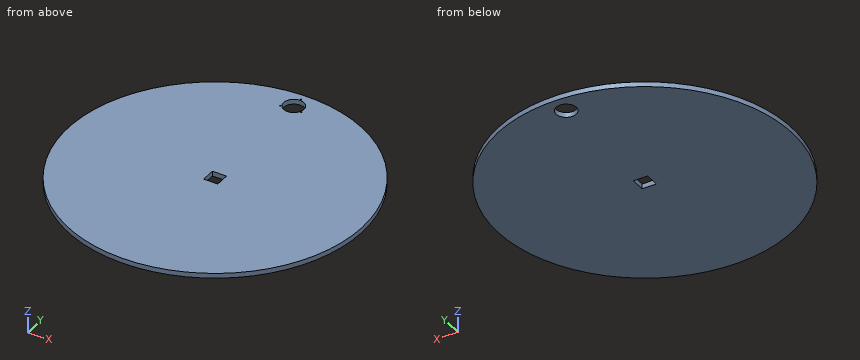
```python
from build123d import *

# Parameters (mm, degrees)
F0_R     = 600
F0_W     = 58.1
F0_H     = 58.1
F1_DEPTH = 20
F3_R     = 41.5
F4_DEPTH = 20.001
F5_D     = 5.1054
F5_DEPTH = 15.81
F5_TIP   = 1.5338169022


with BuildPart() as f1:
    # F0 (on Top) → F1 (new body)
    with BuildSketch(Plane.XY):
        Circle(F0_R)
        Rectangle(F0_W, F0_H, mode=Mode.SUBTRACT)
    extrude(amount=F1_DEPTH)

    # F3 (on offset) → F4 (cut, through all)
    with BuildSketch(Plane.XY.offset(20)):
        with Locations((0.1939173973, 525.9999642548)):
            Circle(F3_R)
    extrude(amount=-F4_DEPTH, mode=Mode.SUBTRACT)

    # F5
    with Locations(Plane.XY.offset(20)):
        with Locations((-40.7258506305, 502.1913310914), (43.0168926358, 505.8476182242), (0.1938496983, 573.0663310914)):
            Hole(F5_D / 2, depth=F5_DEPTH)
            with Locations((0, 0, -(F5_DEPTH + F5_TIP / 2))):  # 118° drill point
                Cone(0, F5_D / 2, F5_TIP, mode=Mode.SUBTRACT)


solid = f1.part
```
Could you check a few things on this model? Use its own coordinates, in mm. Coordinates: 2 decimals unless noted, no trailing zeros. Loops run counter-clockwise (first coordinate to the right, second up) from the corner with the lowest first, then second, coordinate; pieces in that order, holes last. Notation, with made-up numbers: M 88.25,1.25 L 93.25,1.25 A25 cw 93.25,29.25 Z; hole C 71.5,12 d3. An arc over 180 degrees is marked long. Put each result on its own line as item: value. Start each with the question number.
(1) Will these pins go through, and if not, where does the flat tip stop? P1, Ø8, axis at y = -183, z = 11, coming from the -X side; P2, Ø12, axis at x = 427, z = 13.5, coming from the -Y side; P3, Ø1, axis at y = 39.5, z = 15, coming from the +X side.
(2) Suppose I cut it at D-D on y = 373. Please give me the cut outline in (x, z), then the cut area to 3 significant figures.
(3) Suppose I cut it at C-C on x = 163. Please give me the cut outline in (y, z).
(4) Suppose I cut it at B-B on z = 7.25. Please give me the cut outline in (x, y), then the cut area to 3 significant figures.
(5) Suppose I cut it at A-A on y = 0. Please give me the cut outline in (x, z).
(6) I need wall thicknesses on line 1 (X direction, y = 353.5, z = 16.5); line 2 (Y direction, x = -460, z = 17.5). Which ranges of each line are inside material? Lowest first, please. Write a range as from..to.
Solutions:
1. P1: stops at x = -572.68
1. P2: stops at y = -427.5
1. P3: stops at x = 598.73
2. outline: M -469.97,0 L 469.97,0 L 469.97,20 L -469.97,20 Z
2. area: 18,800 mm2
3. outline: M -577.43,0 L 577.43,0 L 577.43,20 L -577.43,20 Z
4. outline: C 0,0 d1200; hole C -40.73,502.19 d5.11; hole C 0.19,526 d83; hole M -29.05,-29.05 L 29.05,-29.05 L 29.05,29.05 L -29.05,29.05 Z; hole C 0.19,573.07 d5.11; hole C 43.02,505.85 d5.11
4. area: 1,120,000 mm2
5. outline: M -600,0 L -29.05,0 L -29.05,20 L -600,20 Z; M 29.05,0 L 600,0 L 600,20 L 29.05,20 Z
6. line 1: x = -484.81..484.81
6. line 2: y = -385.23..385.23
